CAD build for the part. Positions are in the model's coordinates, mm. Face numbers are marked on the shaded views. A direction names the side the tool comes from. Round coordinates to 2 decimals unless told otherwise and drop trailing zeros. Loops run counter-clockwise (first coordinate to the right, second up) from the corner with the lowest first, then second, coordinate; pieces in that order, holes last. Notation, with made-up numbers: M 57,1 L 75,1 A8 ccw 75,11 Z; hole C 22,79 d10. An arc over 180 degrees is marked long. Use a Markdown table: item, result. Add a question column.
(1) Two-plate mould, pull along Y, no slides. Class the marked faces 3, 4 and 5: released by +Y, released by -Y, zero draft, split by the parting line, or undercut.
(2) Which spindle directions (+Z, -Z, +X, -X, +Y, -Y) get a long thin tool onto all of the face, cutting with end or side? Do the marked faces 1 and 2. Say none if no direction does.
(3) Wall check: L1, parallel to Y at x = 0, z = 3.2; L2, parallel to Y at x = 1.75, z = 3; L3, parallel to Y at x = 0, z = -0.5. Give the ranges that are in metal, low to high.
(4) Band-saw the part on A-A, the plane z = 1. Write the cut outline in (x, y).
from build123d import *

# Parameters (mm, degrees)
F0_R     = 11
F0_R_2   = 9
F1_DEPTH = 3.5
F0_R_3   = 6
F0_R_4   = 4
F2_DEPTH = 2.75
F3_SIZE  = 0.1


with BuildPart() as f1:
    # F0 (on Top) → F1 (new body, symmetric)
    with BuildSketch(Plane.XY):
        Circle(F0_R)
        Circle(F0_R_2, mode=Mode.SUBTRACT)
    extrude(amount=F1_DEPTH, both=True)



with BuildPart() as f1b:
    # F0 (on Top) → F1, piece 2 (new body, symmetric)
    with BuildSketch(Plane.XY):
        Circle(F0_R_3)
        Circle(F0_R_4, mode=Mode.SUBTRACT)
    extrude(amount=F1_DEPTH, both=True)


with BuildPart() as f1_1:
    add(f1.part)

    add(f1b.part)  # F2 merges F1b
    # F0 (on Top) → F2 (join, symmetric)
    with BuildSketch(Plane.XY):
        Circle(F0_R_2)
        Circle(F0_R_3, mode=Mode.SUBTRACT)
    extrude(amount=F2_DEPTH, both=True)

    # F3
    f3_edges = [f1_1.edges().sort_by_distance(p)[0] for p in [
        (-4, 0, 3.5),
        (-4, 0, -3.5),
        (-11, 0, 3.5),
        (-9, 0, 3.5),
        (-6, 0, 3.5),
        (-11, 0, -3.5),
        (-9, 0, -3.5),
        (-6, 0, -3.5),
    ]]
    chamfer(f3_edges, length=F3_SIZE)


solid = f1_1.part
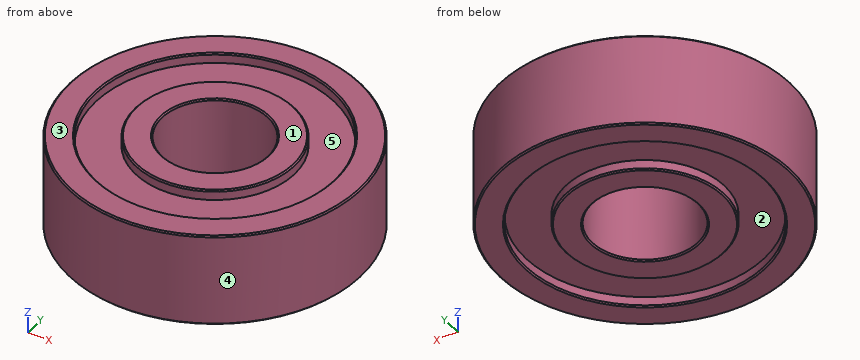
Return value:
| question | item | result |
|---|---|---|
| 1 | face 3 | zero draft |
| 1 | face 4 | split by the parting line |
| 1 | face 5 | undercut |
| 2 | face 1 | +Z, +X, -X, +Y, -Y |
| 2 | face 2 | -Z |
| 3 | L1 | -11 to -9, -6 to -4, 4 to 6, 9 to 11 |
| 3 | L2 | -10.86 to -8.83, -5.74 to -3.6, 3.6 to 5.74, 8.83 to 10.86 |
| 3 | L3 | -11 to -4, 4 to 11 |
| 4 | outline | C 0,0 d22; hole C 0,0 d8 |
